Here's how the part is built. I have some questions about the finished solid (model axes, mm). A direction names the side the tool comes from. Coordinates: 2 decimals unless noted, no trailing zeros. Write each loop counter-clockwise with the first axis right and the second up, starting at its lowest first coordinate (ties: lowest second). Pieces come first, ordered by that corner, then holes. Notation, with made-up numbers: M 41,-39.5 L 100,-39.5 A34 ccw 100,-5.5 Z; hole C 0.5,88 d3. An arc over 180 degrees is marked long. Use a Markdown table: item, result.
```python
from build123d import *

# Parameters (mm, degrees)
BOSS_EXTRUDE1_START     = 80
SKETCH1_R               = 15
BOSS_EXTRUDE1_DEPTH     = 10
SKETCH1_3_R             = 15
BOSS_EXTRUDE2_DEPTH     = 15
BOSS_EXTRUDE3_DEPTH     = 10
BOSS_EXTRUDE4_DEPTH     = 10
SKETCH4_W               = 25
SKETCH4_H               = 10
BOSS_EXTRUDE6_DEPTH     = 60
CUT_EXTRUDE1_DEPTH      = 188.082869339
CUT_EXTRUDE1_DEPTH_BACK = 188.082869339
BOSS_EXTRUDE7_START     = 10
BOSS_EXTRUDE7_DEPTH     = 10


with BuildPart() as part:
    # Sketch1 → Boss-Extrude1 (new body)
    with BuildSketch(Plane(origin=(0, 0, 0), x_dir=(1, 0, 0), z_dir=(0, 1, 0)).offset(BOSS_EXTRUDE1_START)):
        with BuildLine():
            Line((50, 50), (25, 50))
            Line((25, 50), (25, 25))
            Line((25, 25), (-50, 25))
            ThreePointArc((-50, 25), (-75, 0), (-50, -25))
            Line((-50, -25), (-50, -50))
            Line((-50, -50), (-25, -50))
            Line((-25, -50), (-25, -25))
            Line((-25, -25), (50, -25))
            ThreePointArc((50, -25), (75, 0), (50, 25))
            Line((50, 25), (50, 50))
        make_face()
        with Locations(Location((-50, 0, 0), (0, 0, 270))):
            Circle(SKETCH1_R, mode=Mode.SUBTRACT)
        with Locations(Location((50, 0, 0), (0, 0, 270))):
            Circle(SKETCH1_R, mode=Mode.SUBTRACT)
    extrude(amount=BOSS_EXTRUDE1_DEPTH)



with BuildPart() as body_2:
    # Sketch1_3 → Boss-Extrude2 (new body)
    # profile 1 of 3: a face of its own
    with BuildSketch(Plane(origin=(0, 0, 0), x_dir=(1, 0, 0), z_dir=(0, 1, 0))):
        with BuildLine():
            Line((25, 50), (-50, 50))
            ThreePointArc((-50, 50), (-100, 0), (-50, -50))
            Line((-50, -50), (-50, -25))
            ThreePointArc((-50, -25), (-75, 0), (-50, 25))
            Line((-50, 25), (25, 25))
            Line((25, 25), (25, 50))
        make_face()
    # profile 2 of 3: a face of its own
    with BuildSketch(Plane(origin=(0, 0, 0), x_dir=(1, 0, 0), z_dir=(0, 1, 0))):
        with BuildLine():
            Line((50, 50), (25, 50))
            Line((25, 50), (25, 25))
            Line((25, 25), (-50, 25))
            ThreePointArc((-50, 25), (-75, 0), (-50, -25))
            Line((-50, -25), (-50, -50))
            Line((-50, -50), (-25, -50))
            Line((-25, -50), (-25, -25))
            Line((-25, -25), (50, -25))
            ThreePointArc((50, -25), (75, 0), (50, 25))
            Line((50, 25), (50, 50))
        make_face()
        with Locations(Location((-50, 0, 0), (0, 0, 270))):
            Circle(SKETCH1_3_R, mode=Mode.SUBTRACT)
        with Locations(Location((50, 0, 0), (0, 0, 270))):
            Circle(SKETCH1_3_R, mode=Mode.SUBTRACT)
    # profile 3 of 3: a face of its own
    with BuildSketch(Plane(origin=(0, 0, 0), x_dir=(1, 0, 0), z_dir=(0, 1, 0))):
        with BuildLine():
            ThreePointArc((50, -50), (100, 0), (50, 50))
            Line((50, 50), (50, 25))
            ThreePointArc((50, 25), (75, 0), (50, -25))
            Line((50, -25), (-25, -25))
            Line((-25, -25), (-25, -50))
            Line((-25, -50), (50, -50))
        make_face()
    extrude(amount=BOSS_EXTRUDE2_DEPTH)


with BuildPart() as part_1:
    add(part.part)

    add(body_2.part)  # Boss-Extrude3 merges body 2
    # Sketch2 → Boss-Extrude3 (add)
    with BuildSketch(Plane.XY.offset(50)):
        Polygon((50, 15), (-25, 80), (-50, 80), (25, 15), align=None)
    extrude(amount=-BOSS_EXTRUDE3_DEPTH)

    # Sketch3 → Boss-Extrude4 (add)
    with BuildSketch(Plane(origin=(0, 0, -50), x_dir=(-1, 0, 0), z_dir=(0, 0, -1))):
        Polygon((-25, 80), (50, 15), (25, 15), (-50, 80), align=None)
    extrude(amount=-BOSS_EXTRUDE4_DEPTH)

    # Sketch4 → Boss-Extrude6 (add)
    with BuildSketch(Plane(origin=(0, 90, 0), x_dir=(1, 0, 0), z_dir=(0, 1, 0))):
        with BuildLine():
            Line((-25, -50), (50, -50))
            ThreePointArc((50, -50), (100, 0), (50, 50))
            Line((50, 50), (50, 40))
            ThreePointArc((50, 40), (90, 0), (50, -40))
            Line((50, -40), (-25, -40))
            Line((-25, -40), (-25, -50))
        make_face()
        with Locations((37.5, 45)):
            Rectangle(SKETCH4_W, SKETCH4_H)
        with BuildLine():
            ThreePointArc((-50, 50), (-100, 0), (-50, -50))
            Line((-50, -50), (-50, -40))
            ThreePointArc((-50, -40), (-90, 0), (-50, 40))
            Line((-50, 40), (25, 40))
            Line((25, 40), (25, 50))
            Line((25, 50), (-50, 50))
        make_face()
        with Locations((-37.5, -45)):
            Rectangle(SKETCH4_W, SKETCH4_H)
    extrude(amount=BOSS_EXTRUDE6_DEPTH)

    # Sketch6 → Cut-Extrude1 (cut, two sides: drawn at the far end of the back side and taken through both)
    with BuildSketch(Plane.XY.offset(-CUT_EXTRUDE1_DEPTH_BACK)):
        Polygon((-639.560936873, -5.139150907), (-100, 90), (134.669192778, 131.378510228), (674.230129651, 226.517661135), (483.951827837, 1305.639534881), (-829.839238687, 1073.982722839), align=None)
    extrude(amount=CUT_EXTRUDE1_DEPTH + CUT_EXTRUDE1_DEPTH_BACK, mode=Mode.SUBTRACT)

    # Sketch7 → Boss-Extrude7 (add)
    with BuildSketch(Plane.XZ.offset(-90).offset(BOSS_EXTRUDE7_START)):
        with BuildLine():
            Line((50, -50), (-50, -50))
            ThreePointArc((-50, -50), (-85.355339059, -35.355339059), (-100, 0))
            ThreePointArc((-100, 0), (-85.355339059, 35.355339059), (-50, 50))
            Line((-50, 50), (-27.684093833, 50))
            Line((-27.684093833, 50), (50, 50))
            ThreePointArc((50, 50), (100, 0), (50, -50))
        make_face()
        with BuildLine():
            Line((-50, -40), (50, -40))
            ThreePointArc((50, -40), (90, 0), (50, 40))
            Line((50, 40), (-50, 40))
            ThreePointArc((-50, 40), (-90, 0), (-50, -40))
        make_face(mode=Mode.SUBTRACT)
    extrude(amount=-BOSS_EXTRUDE7_DEPTH)


solid = part_1.part
```
1. Suppose I cut it at A-A on z = 35.5. Write out the boundary of the cut face in (x, y).
Answers follow:
| item | result |
|---|---|
| outline | M -85.21,0 L 85.21,0 L 85.21,15 L -85.21,15 Z; M -85.21,80 L -68.43,80 L -68.43,95.57 L -85.21,92.61 Z; M -50,80 L -25,80 L -25,90 L -50,90 Z; M 68.43,80 L 85.21,80 L 85.21,122.66 L 68.43,119.7 Z |
2. Which directions (+Z, -Z, +X, -X, +Y, -Y) give clear straight access to the entire face, cutting with the end or side of a thin tool? Please do faces 4 (the face through (50, 85, -32)), 5 (the face through (-1, 80, -1)), 6 (the face through (-1, 0, -1)).
Answers follow:
| item | result |
|---|---|
| face 4 | +Y |
| face 5 | +X, -X |
| face 6 | +Z, -Z, +X, -X, -Y |
3. Suppose I cut it at B-B on x = -83.5. Write out the boundary of the cut face in (y, z).
Answers follow:
| item | result |
|---|---|
| outline | M 0,-37.12 L 15,-37.12 L 15,37.12 L 0,37.12 Z; M 80,-37.12 L 92.91,-37.12 L 92.91,-21.86 L 80,-21.86 Z; M 80,21.86 L 92.91,21.86 L 92.91,37.12 L 80,37.12 Z |
4. Will these pins go through, and if not, where does the flat tip stop? pin 1 Ø1.5 at (y, z) = (82, -31.5) entering from -X; pin 2 Ø5 at (y, z) = (85.5, 31) entering from -X; pin 3 Ø1.5 at (x, z) = (44, 32) entering from +Y.
Answers follow:
| item | result |
|---|---|
| pin 1 | stops at x = -89.43 |
| pin 2 | stops at x = -91.08 |
| pin 3 | stops at y = 15 |
5. We'd pull the mould along X, two halves only. Please class faces 1 (the face through (0, 50, -40)), 2 (the face through (12, 94, 40)), 3 (the face through (11.98, 47.05, -45.07)): +X half, -X half, draft (parallel to the pull), parting line (faces both ways), or undercut.
Answers follow:
| item | result |
|---|---|
| face 1 | draft |
| face 2 | undercut |
| face 3 | +X half |
6. Suppose I cut it at C-C on x = -20.5. Write out the boundary of the cut face in (y, z), and give its area (3 significant figures).
Answers follow:
| item | result |
|---|---|
| outline | M 0,-50 L 15,-50 L 15,50 L 0,50 Z; M 18.9,-50 L 40.57,-50 L 40.57,-40 L 18.9,-40 Z; M 54.43,40 L 76.1,40 L 76.1,50 L 54.43,50 Z; M 80,-50 L 104.02,-50 L 104.02,-40 L 80,-40 Z; M 80,-25 L 90,-25 L 90,25 L 80,25 Z; M 80,40 L 104.02,40 L 104.02,50 L 80,50 Z |
| area | 2,910 mm2 |
7. I need wall thicknesses on probe 1 along X at (y, z) = (9, 0); probe 2 along X at (y, z) = (88.25, 0); probe 3 along Y at (x, z) = (42, 20.5). Which ranges of each line are inside material? Lowest first, please.
Answers follow:
| item | result |
|---|---|
| probe 1 | x = -100 to -65, -35 to 35, 65 to 100 |
| probe 2 | x = -100 to -90, -75 to -65, -35 to 35, 65 to 75, 90 to 100 |
| probe 3 | y = 0 to 15, 80 to 90 |
